Part model, mm, in its own coordinate system. A direction names the side the tool comes from. Round coordinates to 2 decimals unless told otherwise and drop trailing zeros. Loops run counter-clockwise (first coordinate to the right, second up) from the corner with the lowest first, then second, coordinate; pieces in that order, holes last. Notation, with made-up numbers: (-10, 70.25) - (21, 70.25) arc R22 cw to (21, 85.25) - close; hole circle Ø6 at (-2.75, 30). An arc over 180 degrees is marked (long way). Write each question's results on one line, items separated by ' | '. Start each with the question number.
(1) Drill centre lines: L1, parallel to Z at x = 0.85, y = 0.15; L2, parallel to X at y = -0.5, z = -8; L3, parallel to X at y = -0.1, z = -5. Where is each one in solid material? Low to high.
(2) Cut at B-B, the plane y = 0. List the corners of the cut face in (x, z), then the cut area to 3 significant figures.
(3) Mould opens along Y. For faces 4 (the face through (0, -0.5, -10)), 5 (the face through (0, 0, 4.9)), 6 (the face through (-0.03, -1.64, -10.96)) say: released by +Y, released by -Y, zero draft, split by the parting line, or undercut.
(4) Cut at A-A, the plane x = 0. List the corners of the cut face in (y, z).
(5) Cut at D-D, the plane z = 2. List the corners of the cut face in (x, y).
(6) Flat gauge pins, fed straight in: P1, Ø1.5, axis at x = -1, z = 2.5, coming from the -Y side; P2, Ø1, axis at x = 1.5, y = 1.5, coming from the -Z side; P3, Ø0.5, axis at x = -1, z = -10, coming from the -Y side. Where does each tip first touch, or does it go through?
(7) Tool access for faces 1 (the face through (0, 0.5, -10)), 2 (the face through (-1.216, 1.115, 2.169)), 3 (the face through (1.847, -0.766, -5.226)): list every direction of +Z, -Z, +X, -X, +Y, -Y with a clear straight run to the whole face (end or side of a thin tool).
(8) Cut at C-C, the plane z = -0.25. List the corners of the cut face in (x, y).
from build123d import *

# Parameters (mm, degrees)
F0_R     = 1.65
F1_DEPTH = 4.9
F0_R_2   = 2
F2_DEPTH = 11.1
F3_SIZE  = 0.5
F4_W     = 4
F4_H     = 1
F5_DEPTH = 1.5
F6_SIZE  = 0.5


with BuildPart() as f1:
    # F0 (on Top) → F1 (new body)
    with BuildSketch(Plane.XY):
        Circle(F0_R)
    extrude(amount=F1_DEPTH)

    # F0 (on Top) → F2 (join)
    with BuildSketch(Plane.XY):
        Circle(F0_R_2)
        Circle(F0_R, mode=Mode.SUBTRACT)
        Circle(F0_R)
    extrude(amount=-F2_DEPTH)

    # F3
    f3_edges = [f1.edges().sort_by_distance(p)[0] for p in [
        (-1.65, 0, 4.9),
        (-2, 0, -11.1),
    ]]
    chamfer(f3_edges, length=F3_SIZE)

    # F4 (on face) → F5 (cut)
    with BuildSketch(Plane(origin=(0, 0, -11.1), x_dir=(1, 0, 0), z_dir=(0, 0, -1))):
        Rectangle(F4_W, F4_H)
    extrude(amount=-F5_DEPTH, mode=Mode.SUBTRACT)

    # F6
    f6_edges = [f1.edges().sort_by_distance(p)[0] for p in [
        (0, 0.5, -11.1),
        (0, -0.5, -11.1),
    ]]
    chamfer(f6_edges, length=F6_SIZE)


solid = f1.part
A:
1) L1: -9.6 to 4.9 | L2: -1.94 to 1.94 | L3: -2 to 2
2) outline: (-2, -9.6) - (2, -9.6) - (2, 0) - (1.65, 0) - (1.65, 4.4) - (1.15, 4.9) - (-1.15, 4.9) - (-1.65, 4.4) - (-1.65, 0) - (-2, 0) - close | area: 54.3 mm2
3) face 4: undercut | face 5: zero draft | face 6: released by -Y
4) outline: (-2, -10.6) - (-1.5, -11.1) - (-1, -11.1) - (-0.5, -10.6) - (-0.5, -9.6) - (0.5, -9.6) - (0.5, -10.6) - (1, -11.1) - (1.5, -11.1) - (2, -10.6) - (2, 0) - (1.65, 0) - (1.65, 4.4) - (1.15, 4.9) - (-1.15, 4.9) - (-1.65, 4.4) - (-1.65, 0) - (-2, 0) - close
5) outline: circle Ø3.3 at (0, 0)
6) P1: y = -1.63 | P2: z = -10.98 | P3: y = -1.85
7) face 1: -Z, +X, -X | face 2: +Z | face 3: +Z, -Z
8) outline: circle Ø4 at (0, 0)
